Here's how the part is built. I have some questions about the finished solid (model axes, mm). Round coordinates to 2 decimals unless told otherwise and drop trailing zeros. Write each loop counter-clockwise with the first axis right and the second up, starting at its lowest first coordinate (ties: lowest second). Pieces come first, ordered by that corner, then holes. Notation, with made-up numbers: (32, 25) -> (76, 25) arc R10 ccw to (76, 41) -> close; hole circle Ø10 at (60.5, 83.5). An arc over 180 degrees is marked (long way). Put each result on its own line as item: value. Start each with the question number.
1) Will this pin go through, and if not, where does the flat tip stop? P1, Ø4, axis at x = 0, y = 22, coming from the +Z side (3 decimals).
2) We'd pull the mould along Y, two halves only. Please class faces 1 (the cylindrical face through (-20.35, 0.07, -2.72)), 2 (the flat face through (0, -35, -2)), 3 (the flat face through (15, 0, 0)), 4 (the cylindrical face through (-22.284, 24.615, -2.72)): released by +Y, released by -Y, zero draft, split by the parting line, or undercut.
3) I want a section at C-C, the plane x = -9. List the corners of the cut face in (y, z) for me.
4) I want a section at B-B, the plane z = -3.9. Give the number of separate pieces and of enclosed holes in the cut face, then the cut area to 3 significant figures.
5) If I drill on line 1 along Y through (x, z) = (0, -2.4); line 2 along Y through (x, z) = (22, -2.15), over which ranges is the centre line in solid material (lowest first)? Write a range as [from, to].
6) I want a section at A-A, the plane y = 0. List the corners of the cut face in (x, z) for me (3 decimals).
from build123d import *

# Parameters (mm, degrees)
SKETCH1_W                       = 70
SKETCH1_H                       = 70
SKETCH1_R                       = 12.5
BASE_FLANGE1_DEPTH              = 5
M4X0_7_TAPPED_HOLE1_D           = 3.3
M4X0_7_TAPPED_HOLE1_DEPTH       = 10.1
M4X0_7_TAPPED_HOLE1_CSINK_D     = 4.05
M4X0_7_TAPPED_HOLE1_CSINK_ANGLE = 90
M4X0_7_TAPPED_HOLE1_TIP         = 0.991420021
M4X0_7_TAPPED_HOLE2_D           = 3.3
M4X0_7_TAPPED_HOLE2_DEPTH       = 10.1
M4X0_7_TAPPED_HOLE2_CSINK_D     = 4.05
M4X0_7_TAPPED_HOLE2_CSINK_ANGLE = 90
M4X0_7_TAPPED_HOLE2_TIP         = 0.991420021
FILLET1_R                       = 10


# Sheet-metal steps are written as plain solids
with BuildPart() as part:
    # Sketch1 → Base-Flange1 (new body)
    with BuildSketch(Plane.XY):
        Rectangle(SKETCH1_W, SKETCH1_H)
        Circle(SKETCH1_R, mode=Mode.SUBTRACT)
    extrude(amount=-BASE_FLANGE1_DEPTH)

    # M4x0.7 Tapped Hole1
    with Locations(Plane.XY):
        with Locations((0, 22), (-22, 0), (0, -22), (22, 0)):
            CounterSinkHole(M4X0_7_TAPPED_HOLE1_D / 2, M4X0_7_TAPPED_HOLE1_CSINK_D / 2, depth=M4X0_7_TAPPED_HOLE1_DEPTH, counter_sink_angle=M4X0_7_TAPPED_HOLE1_CSINK_ANGLE)
            with Locations((0, 0, -(M4X0_7_TAPPED_HOLE1_DEPTH + M4X0_7_TAPPED_HOLE1_TIP / 2))):  # 118° drill point
                Cone(0, M4X0_7_TAPPED_HOLE1_D / 2, M4X0_7_TAPPED_HOLE1_TIP, mode=Mode.SUBTRACT)

    # M4x0.7 Tapped Hole2
    with Locations(Plane.XY):
        with Locations((-23.5, 23.5), (23.5, 23.5), (23.5, -23.5), (-23.5, -23.5)):
            CounterSinkHole(M4X0_7_TAPPED_HOLE2_D / 2, M4X0_7_TAPPED_HOLE2_CSINK_D / 2, depth=M4X0_7_TAPPED_HOLE2_DEPTH, counter_sink_angle=M4X0_7_TAPPED_HOLE2_CSINK_ANGLE)
            with Locations((0, 0, -(M4X0_7_TAPPED_HOLE2_DEPTH + M4X0_7_TAPPED_HOLE2_TIP / 2))):  # 118° drill point
                Cone(0, M4X0_7_TAPPED_HOLE2_D / 2, M4X0_7_TAPPED_HOLE2_TIP, mode=Mode.SUBTRACT)

    # Fillet1
    fillet1_edges = [part.edges().sort_by_distance(p)[0] for p in [
        (35, -35, -2.5),
        (-35, -35, -2.5),
        (-35, 35, -2.5),
        (35, 35, -2.5),
    ]]
    fillet(fillet1_edges, radius=FILLET1_R)


solid = part.part
Findings:
1. P1: stops at z = -0.025
2. face 1: undercut
2. face 2: released by -Y
2. face 3: zero draft
2. face 4: undercut
3. outline: (-35, -5) -> (-8.67, -5) -> (-8.67, 0) -> (-35, 0) -> close; (8.67, -5) -> (35, -5) -> (35, 0) -> (8.67, 0) -> close
4. separate pieces: 1
4. enclosed holes: 9
4. area: 4,250 mm2
5. line 1: y = [-35, -23.65], [-20.35, -12.5], [12.5, 20.35], [23.65, 35]
5. line 2: y = [-35, -24.19], [-22.81, -1.65], [1.65, 22.81], [24.19, 35]
6. outline: (-35, -5) -> (-23.65, -5) -> (-23.65, -0.375) -> (-24.025, 0) -> (-35, 0) -> close; (-20.35, -5) -> (-12.5, -5) -> (-12.5, 0) -> (-19.975, 0) -> (-20.35, -0.375) -> close; (12.5, -5) -> (20.35, -5) -> (20.35, -0.375) -> (19.975, 0) -> (12.5, 0) -> close; (23.65, -5) -> (35, -5) -> (35, 0) -> (24.025, 0) -> (23.65, -0.375) -> close
